```python
from build123d import *

# Parameters (mm, degrees)
F1_DEPTH = 54.5
F2_W     = 11
F2_H     = 8
F3_DEPTH = 17.5
F4_START = -9.5
F4_DEPTH = 17.7


with BuildPart() as f1:
    # F0 (on Top) → F1 (new body, symmetric)
    with BuildSketch(Plane.XY):
        with BuildLine():
            Line((-15, -25.9807621135), (-13.8452994616, -25.9807621135))
            Line((-13.8452994616, -25.9807621135), (-7.7845367167, -15.4832131067))
            ThreePointArc((-7.7845367167, -15.4832131067), (-8.2281965887, -15.2520713642), (-8.665, -15.0082202476))
            Line((-8.665, -15.0082202476), (-15, -25.9807621135))
        make_face()
        with BuildLine():
            Line((-13.8452994616, -25.9807621135), (0, -25.9807621135))
            Line((0, -25.9807621135), (0, -17.33))
            ThreePointArc((0, -17.33), (-4.0003010425, -16.8619836191), (-7.7845367167, -15.4832131067))
            Line((-7.7845367167, -15.4832131067), (-13.8452994616, -25.9807621135))
        make_face()
        with BuildLine():
            Line((0, -25.9807621135), (1, -25.9807621135))
            Line((1, -25.9807621135), (1, -17.3011242409))
            ThreePointArc((1, -17.3011242409), (0.5002084089, -17.3227795561), (0, -17.33))
            Line((0, -17.33), (0, -25.9807621135))
        make_face()
        with BuildLine():
            Line((1, -25.9807621135), (15, -25.9807621135))
            Line((15, -25.9807621135), (8.665, -15.0082202476))
            ThreePointArc((8.665, -15.0082202476), (4.9666294839, -16.6030566936), (1, -17.3011242409))
            Line((1, -17.3011242409), (1, -25.9807621135))
        make_face()
    extrude(amount=F1_DEPTH, both=True)

    # F2 (on Right) → F3 (cut, symmetric)
    with BuildSketch(Plane.YZ):
        with Locations((-19.4807621135, 49.5)):
            Rectangle(F2_W, F2_H)
        with Locations((-19.4807621135, 40.5)):
            Rectangle(F2_W, F2_H)
        with Locations((-19.4807621135, 31.5)):
            Rectangle(F2_W, F2_H)
        with Locations((-19.4807621135, 22.5)):
            Rectangle(F2_W, F2_H)
        with Locations((-19.4807621135, 13.5)):
            Rectangle(F2_W, F2_H)
        with Locations((-19.4807621135, 4.5)):
            Rectangle(F2_W, F2_H)
        with Locations((-19.4807621135, -4.5)):
            Rectangle(F2_W, F2_H)
        with Locations((-19.4807621135, -13.5)):
            Rectangle(F2_W, F2_H)
        with Locations((-19.4807621135, -22.5)):
            Rectangle(F2_W, F2_H)
        with Locations((-19.4807621135, -31.5)):
            Rectangle(F2_W, F2_H)
        with Locations((-19.4807621135, -40.5)):
            Rectangle(F2_W, F2_H)
        with Locations((-19.4807621135, -49.5)):
            Rectangle(F2_W, F2_H)
    extrude(amount=F3_DEPTH, both=True, mode=Mode.SUBTRACT)

    # F0 (on Top) → F4 (join)
    with BuildSketch(Plane.XY.offset(F4_START)):
        with BuildLine():
            Line((0, -25.9807621135), (1, -25.9807621135))
            Line((1, -25.9807621135), (1, -17.3011242409))
            ThreePointArc((1, -17.3011242409), (0.5002084089, -17.3227795561), (0, -17.33))
            Line((0, -17.33), (0, -25.9807621135))
        make_face()
    extrude(amount=-F4_DEPTH)


solid = f1.part
```
The model under review builds one solid part; all positions refer to its coordinate system, in mm. A direction names the side the tool comes from. Coordinates: 2 decimals unless noted, no trailing zeros. Write each loop counter-clockwise with the first axis right and the second up, starting at its lowest first coordinate (ties: lowest second). Pieces come first, ordered by that corner, then holes. Notation, with made-up numbers: (-39, 89.5) - (0, 89.5) arc R28 ccw to (0, 115.5) - close; hole circle Ø2 at (-26, -27.75). An arc over 180 degrees is marked (long way). Answer in a Markdown table with one row per item. Add a question column.
Q1. Consider section C-C on z = 38. Give the boundary of the cut face in (x, y), then the cut area to 3 significant figures.
Q2. To check wall thickness, follow line 1 along Y through (x, z) = (-9.75, -26); line 2 along X through (y, z) = (-22, -11); line 3 along X through (y, z) = (-15.75, -36). State the ranges of each line that lie inside material, in increasing order. Write a range as from..to.
Q3. Clearance check with flat-ended pins moving along their axes: pin 1 (9 mm diameter, centred on x = -4.5, z = 3.5, fed in from +Y); pin 2 (4 mm diameter, centred on x = -8.5, z = -12, fed in from +Y); pin 3 (6 mm diameter, centred on y = -19.5, z = -39, fed in from +X). State where each tip first meets the part, or that it passes through.
Q4. For faces 4 (the face through (0, -21, -13)), 5 (the face through (0, -24.981, -5)), 6 (the face through (8, -24.981, -14)), list the 3-axis set-ups (+Z, -Z, +X, -X, +Y, -Y) from which the entire face can be reached by the end or side of a thin tool; tool diameter is ignored.
Q5. Draft analysis for pull direction Z (two halves, no side actions). For faces 1 (the face through (0, -22, 54.5)), 2 (the face through (0, -22, -54.5)), 3 (the face through (1, -21, -22)), state which applies: +Z half, -Z half, draft (parallel to the pull), parting line (faces both ways), or undercut.
Q6. Consider section A-A on z = -22. Give the boundary of the cut face in (x, y).
Q7. Consider section B-B on y = -21.25. Give the number of separate pieces and of enclosed holes in the cut face, then the cut area to 3 significant figures.
Answers below:
| question | item | result |
|---|---|---|
| 1 | outline | (-15, -25.98) - (15, -25.98) - (14.42, -24.98) - (-14.42, -24.98) - close |
| 1 | area | 29.4 mm² |
| 2 | line 1 | -25.98..-24.98 |
| 2 | line 2 | 0..1 |
| 2 | line 3 | -9.09..-7.23, 7.23..9.09 |
| 3 | pin 1 | y = -15.45 |
| 3 | pin 2 | y = -24.98 |
| 3 | pin 3 | x = 12.22 |
| 4 | face 4 | -X, +Y |
| 4 | face 5 | +X, -X, +Y |
| 4 | face 6 | +X, +Y |
| 5 | face 1 | +Z half |
| 5 | face 2 | -Z half |
| 5 | face 3 | undercut |
| 6 | outline | (-15, -25.98) - (15, -25.98) - (14.42, -24.98) - (1, -24.98) - (1, -17.3) arc R17.33 cw to (0, -17.33) - (0, -24.98) - (-14.42, -24.98) - close |
| 7 | separate pieces | 11 |
| 7 | enclosed holes | 0 |
| 7 | area | 335 mm² |
